Input: part model. Units: mm. Frame: model coordinates. Face numbers are marked on the shaded views. A direction names the side the tool comes from. Coordinates: 2 decimals unless noted, no trailing zeros. Order: outer loops, then holes, each group sorted by start corner. A loop starts at its lowest first (then second) coordinate and runs counter-clockwise, first axis right, second up. Notation, with made-up numbers: (-9.75, 67) -> (40.25, 67) arc R17 ccw to (40.25, 91) -> close; hole circle Ø8 at (-37, -12.75). An arc over 180 degrees is marked (long way). Answer as CSV lines item,"result".
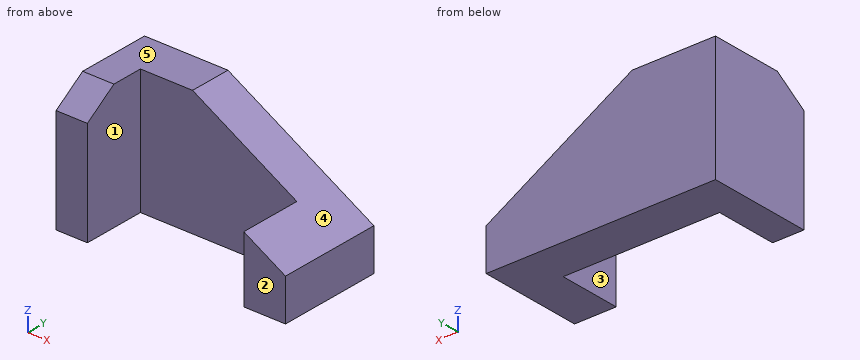
from build123d import *

# Parameters (mm, degrees)
F1_DEPTH = 60
F3_DEPTH = 15
F5_DEPTH = 50


with BuildPart() as f1:
    # F0 (on Top) → F1 (new body)
    with BuildSketch(Plane.XY):
        Polygon((55, 25), (-55, 25), (-55, -25), (-40, -25), (-40, 5), (35, 5), (35, -25), (55, -25), align=None)
    extrude(amount=F1_DEPTH)

    # F2 (on face) → F3 (cut)
    with BuildSketch(Plane.YZ.offset(-40)):
        Polygon((-10, 60), (-25, 60), (-25, 49.899567), align=None)
    extrude(amount=-F3_DEPTH, mode=Mode.SUBTRACT)

    # F4 (on face) → F5 (cut)
    with BuildSketch(Plane(origin=(0, 25, 0), x_dir=(-1, 0, 0), z_dir=(0, 1, 0))):
        Polygon((-55, 20), (15, 60), (-55, 60), align=None)
    extrude(amount=-F5_DEPTH, mode=Mode.SUBTRACT)


solid = f1.part
1. Cut plane D-D (z = 17). Return the cut outline in (x, y).
Findings:
outline,"(-55, -25) -> (-40, -25) -> (-40, 5) -> (35, 5) -> (35, -25) -> (55, -25) -> (55, 25) -> (-55, 25) -> close"
2. Ray query, line 1 along X through (y, z) = (4.5, 9); line 2 along X through (y, z) = (-14.5, 52); line 3 along Y through (x, z) = (-17, 55). Return the intervals inside material, ascending.
Findings:
line 1,"x = -55 to -40, 35 to 55"
line 2,"x = -55 to -40"
line 3,"y = 5 to 25"
3. Cut plane C-C (y = 10.5). Return the cut outline in (x, z).
Findings:
outline,"(-55, 0) -> (55, 0) -> (55, 20) -> (-15, 60) -> (-55, 60) -> close"
4. Reachability of the marked faces 1 and 2 from +Z, -Z, +X, -X, +Y, -Y: full face, straight path, thin tool, end or side. Return the list, or none.
Findings:
face 1,"+Z, -Z, -Y"
face 2,"+Z, -Z, +X, -X, -Y"
5. Contact query for flat-ended pins moving along their axis: pin 1 (10 mm diameter, centred on x = 24.5, z = 27, fed in from -Y); pin 2 (1 mm diameter, centred on x = 42.5, y = 6.5, fed in from +Z); pin 3 (12 mm diameter, centred on x = 5, y = 15.5, fed in from +Z). Output: stop coordinate, or through.
Findings:
pin 1,"stops at y = 5"
pin 2,"stops at z = 27.43"
pin 3,"stops at z = 52"
6. Mould query, pull axis X, two halves, no side actions, for the marked faces 3, 4 and 5. Classes: released by +X, released by -X, zero draft, split by the parting line, or undercut.
Findings:
face 3,"undercut"
face 4,"released by +X"
face 5,"zero draft"
7. Cut plane B-B (z = 24). Return the cut outline in (x, y), plus the area to 3 significant figures.
Findings:
outline,"(-55, -25) -> (-40, -25) -> (-40, 5) -> (35, 5) -> (35, -25) -> (48, -25) -> (48, 25) -> (-55, 25) -> close"
area,"2,900 mm2"
8. Cut plane A-A (y = -7). Return the cut outline in (x, z), plus the area to 3 significant figures.
Findings:
outline,"(-55, 0) -> (-40, 0) -> (-40, 60) -> (-55, 60) -> close; (35, 0) -> (55, 0) -> (55, 20) -> (35, 31.43) -> close"
area,"1,410 mm2"
